Autodesk Inventor part; units mm, degrees
ref_plane "YZ Plane" through (0, 0, 0) normal (1, 0, 0) x (0, 1, 0)
ref_plane "XZ Plane" through (0, 0, 0) normal (0, 1, 0) x (-1, 0, 0)
ref_plane "XY Plane" through (0, 0, 0) normal (0, 0, 1) x (1, 0, 0)
sketch "スケッチ1" plane through (0, 0, 0) normal (1, 0, 0) x (0, 1, 0)
  line L0 (0, 0) -> (0, 6)
  line L1 (0, 6) -> (0, -6)
  line L2 (0, 0) -> (11.5, 0)
  line L3 (11.5, 0) -> (11.5, 9.5)
  line L4 (11.5, 9.5) -> (11.5, -9.5)
  circle A0 centre (0, 6) radius 1.25
  circle A1 centre (0, -6) radius 1.25
  circle A2 centre (11.5, 9.5) radius 1.65
  circle A3 centre (11.5, -9.5) radius 1.65
  circle A4 centre (11.5, 9.5) radius 2.5
  circle A5 centre (11.5, -9.5) radius 2.5
  circle A6 centre (0, 0) radius 2.65
  line L5 (0, 0) -> (-14.6, 0)
  circle A7 centre (-14.6, 0) radius 1.65
  circle A8 centre (-14.6, 0) radius 2.5
  circle A9 centre (0, 6) radius 2
  circle A10 centre (0, -6) radius 2
  line L6 (0, 8) -> (10.6499, 11.851)
  line L7 (0, -8) -> (10.6499, -11.851)
  line L8 (-14.6, 0) -> (-14.6, -2.5)
  line L9 (-14.6, 0) -> (-12.1, 0) construction
  line L10 (-14.6, -2.5) -> (-14.6, 2.5)
  line L11 (-14.6, -2.5) -> (-0.7212, -7.8655)
  line L12 (-14.6, 2.5) -> (-0.7212, 7.8655)
  circle A11 centre (11.5, -9.5) radius 14.9164
  line L13 (11.5, -9.5) -> (0, 0)
  line L14 (11.5, -9.5) -> (0, -2.65)
  line L15 (14, 9.5) -> (14, 6.6979)
  circle A12 centre (11.5, -9.5) radius 16.7294
  circle A13 centre (11.5, -9.5) radius 2.6
  circle A14 centre (11.5, -9.5) radius 16.5
  line L16 (14, 6.6979) -> (14.1, -9.4839)
  line L17 (8.9, -9.5) -> (8.9, 0)
  line L18 (9, 9.5) -> (9, 0)
  line L19 (14.0414, 0) -> (11.5, 0)
  line L20 (2.65, 0) -> (2.65, -4.2285)
  point P0 (9.3522, -8.2206)
  point P1 (0, 2.65)
  point P2 (12.4812, 7.2006)
  point P3 (14, 6.8095)
  point P4 (0.3158, 2.6311)
  point P5 (9.2662, -8.1695)
  dimension "d9" = 5
  dimension "d0" = 6
  dimension "d1" = 12
  dimension "d2" = 11.5
  dimension "d3" = 9.5
  dimension "d4" = 19
  dimension "d5" = 2.5
  dimension "d6" = 3.3
  dimension "d7" = 3.3
  dimension "d8" = 5
  dimension "d10" = 5.3
  dimension "d11" = 14.6
  dimension "d12" = 3.3
  dimension "d13" = 5
  dimension "d14" = 4
  dimension "d15" = 4
  dimension "d16" = 90
  dimension "d21" = 5.2
  dimension "d22" = 33
extrude "押し出し3" add sketch "スケッチ1" along normal blind 3 contours A6 A11 L18 L2 | L2 L17 L13 L20 | A6 A14 L18 A11 | L20 L13 L17 L14 | L2 L4 A13 L13 L17 | L18 A14 L3 A11 | A11 L3 L2 L18 | L17 L13 A13 L14 | A11 L16 L19 L3 | L3 A14 L15 L16 A11 | L19 L16 A13 L4
extrude "押し出し4" add sketch "スケッチ1" against normal blind 2 contours L2 L4 A13 L13 L17 | L17 L13 A13 L14 | L14 A13 L17 | A13 L13 A5 L14 | L14 A5 L7 A13 | L19 L16 A13 L4 | A13 L4 A5 L13 | L7 A5 L4 A13 | L14 A3 L4 A5 | A5 L13 A3 L14 | A5 L4 A3 L13
sketch "スケッチ2" plane through (3, 0, 0) normal (1, 0, 0) x (0, 0, -1)
  line L0 (0, 0) -> (0, 11.4707)
  line L1 (0, 14.0414) -> (0, 8.9)
  line L2 (0, 11.4707) -> (-9.5, 11.4707)
  circle A0 centre (-9.5, 11.4707) radius 1.65
  circle A1 centre (-9.5, 11.4707) radius 2.5
  line L3 (-9.5186, 8.9708) -> (0, 8.9)
  line L4 (0, 11.4707) -> (0, 14.0414)
  line L5 (0, 14.0414) -> (-6.6979, 14)
  line L6 (0, 14.0414) -> (-9.5186, 13.9706)
  line L7 (-9.5, 11.4707) -> (-6.8033, 8.9506)
  line L8 (-9.5, 11.4707) -> (-12, 11.4707)
  line L9 (0, 8.9) -> (7.9513, 8.9)
  line L10 (-9.5, 11.4707) -> (-10.75, 9.3056)
  point P0 (-11.15, 11.4707)
  point P1 (-8.2945, 10.3441)
  point P2 (-10.325, 10.0417)
  dimension "d27" = 9.5
  dimension "d28" = 3.3
  dimension "d29" = 5
extrude "押し出し5" add sketch "スケッチ2" along normal blind 2 contours L3 L7 A1 L2 L0 | L2 A1 L6 L1 | A1 L7 A0 L2 | L2 A0 L8 A1 | A1 L8 A0 L10
properties part number "ikafly2c"
Geometry: final body of the model. Coordinates: model frame, mm. A direction names the side the tool comes from. Coordinates: 2 decimals unless noted, no trailing zeros. Order: outer loops, then holes, each group sorted by start corner. A loop starts at its lowest first (then second) coordinate and runs counter-clockwise, first axis right, second up.
1) Section D-D (y = 7.5). Return loops of the section in (x, z), then the cut area to 3 significant figures.
Result sheet:
outline: (0, -7.12) - (3, -7.12) - (3, 6.51) - (0, 6.51) - close
area: 40.9 mm2
2) Ray query, probe 1 along Y at (x, z) = (-1.2, -9.5); probe 2 along Z at (x, y) = (-0.65, 11.5); probe 3 along X at (y, z) = (7.75, -6). Return the intervals inside material, ascending.
Result sheet:
probe 1: y = 8.9 to 9.85, 13.15 to 14.1
probe 2: z = -12.1 to -11.15, -7.85 to 0
probe 3: x = 0 to 3
3) Section A-A (x = 4.75). Return loops of the section in (y, z) (3 decimals).
Result sheet:
outline: (8.9, 0) - (14.041, 0) - (13.971, 9.519) arc R2.5 ccw to (9.306, 10.75) - (10.042, 10.325) arc R1.65 cw (long way) to (10.344, 8.294) - (8.951, 6.803) - close
4) First-contact query: P1, Ø3, axis at x = -1, z = -6, coming from the +Y side; P2, Ø0.6, axis at x = -1, y = 11, coming from the +Z side; P3, Ø4.5, axis at y = 11.47, z = 9.5, coming from the +X side; P4, Ø4, axis at x = 1, y = 5.5, coming from the +Z side. Flat tips, straight axial feed; report the tip coordinate or a pass-through.
Result sheet:
P1: stops at y = 14.09
P2: stops at z = 0
P3: stops at x = 5
P4: stops at z = 6.51
5) Set-up query: faces 5 (the flat face through (4, 11, 0)), 6 (the flat face through (3.99, 9.66, 7.56)), 7 (the flat face through (-1, 8.9, -5)), 8 (the flat face through (5, 12, 5)), 9 (the cylindrical face through (3.986, 13.093, 9.799)). Return all of +Z, -Z, +X, -X, +Y, -Y with unobstructed straight access to the full face (end or side cutting, diameter ignored); none if empty.
Result sheet:
face 5: -Z, +X, +Y, -Y
face 6: +X, -X, -Y
face 7: +Z, -Z, -X, -Y
face 8: +Z, -Z, +X, +Y, -Y
face 9: +X, -X
6) Section B-B (y = 11.5). Return loops of the section in (x, z).
Result sheet:
outline: (-2, -12.1) - (0, -12.1) - (0, -11.15) - (-2, -11.15) - close; (-2, -7.85) - (0, -7.85) - (0, -6.9) - (3, -6.9) - (3, 0) - (5, 0) - (5, 7.85) - (3, 7.85) - (3, 7) - (0, 7) - (0, 0) - (-2, 0) - close; (3, 11.15) - (5, 11.15) - (5, 12) - (3, 12) - close
7) Draft query along Z for faces 1 (the cylindrical face through (-0.986, 13.024, -10.132)), 2 (the flat face through (0, 7, 1)), 3 (the cylindrical face through (1.479, 1.964, 1.779)), 4 (the flat face through (-1, 11, 0)). Return one class per face: released by +Z, released by -Z, zero draft, split by the parting line, or undercut.
Result sheet:
face 1: undercut
face 2: zero draft
face 3: released by -Z
face 4: released by +Z
